Input: part model. Units: mm. Frame: model coordinates. Face numbers are marked on the shaded views. A direction names the side the tool comes from. Coordinates: 2 decimals unless noted, no trailing zeros. Write each loop counter-clockwise with the first axis right and the second up, starting at its lowest first coordinate (ties: lowest second). Pieces come first, ordered by that corner, then holes.
1) Section query D-D (y = -5). Output: boundary loops of the cut face in (x, z).
2) Section query B-B (x = -16.5). Output: boundary loops of the cut face in (y, z) (3 decimals).
3) Section query A-A (z = 0). Output: boundary loops of the cut face in (x, y), then the cut area to 3 significant figures.
4) Line query: L1, parallel to X at y = -50, z = 9.25; L2, parallel to Y at x = -9, z = 0; L3, parallel to X at y = -26, z = 4. Output: solid intervals per line, ascending.
5) Draft query along Z for the marked faces 1, 2 and 3. Return one class per face: pulls with the +Z half, pulls with the -Z half, needs draft (parallel to the pull), parting line crosses it, or undercut.
6) Pin query (flat end, axial travel): pin 1 Ø8 at (y, z) = (10, -2.5) entering from -X; pin 2 Ø12 at (y, z) = (-28.5, 0.5) entering from +X; pin 3 Ø10 at (y, z) = (14.5, 1.5) entering from +X; pin 4 Ø3 at (y, z) = (-20, -3) entering from -X. Return the tip coordinate at first contact, or that it passes through.
7) Set-up query: the marked faces 4, 5 and 6. Return all of +Z, -Z, +X, -X, +Y, -Y with unobstructed straight access to the full face (end or side cutting, diameter ignored); none if empty.
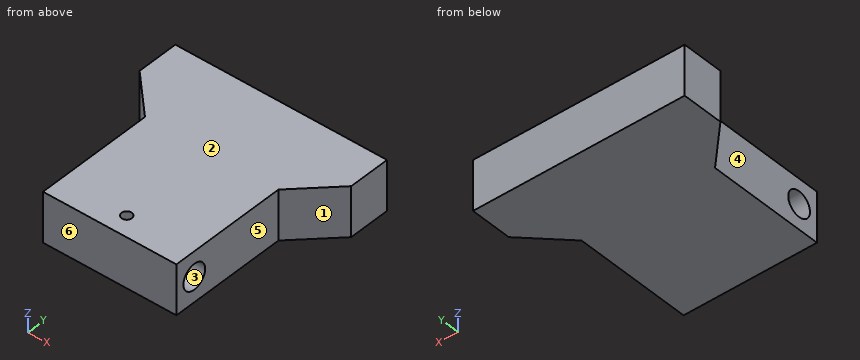
Autodesk Inventor part; units mm, degrees
ref_plane "YZ Plane" through (0, 0, 0) normal (1, 0, 0) x (0, 1, 0)
ref_plane "XZ Plane" through (0, 0, 0) normal (0, 1, 0) x (-1, 0, 0)
ref_plane "XY Plane" through (0, 0, 0) normal (0, 0, 1) x (1, 0, 0)
sketch "Esboço1" plane through (0, 0, 0) normal (0, 0, 1) x (1, 0, 0)
  line L0 (0, 36.3068) -> (0, -8.6932) construction
  circle A0 centre (0, -8.6932) radius 68 construction
  line L1 (0, 36.3068) -> (50.9804, 36.3068)
  line L2 (50.9804, 36.3068) -> (50.9804, 16.3068)
  line L3 (50.9804, 16.3068) -> (32.1355, -2.5381)
  line L4 (32.1355, -2.5381) -> (32.1355, -59.5381)
  line L5 (32.1355, -59.5381) -> (0, -59.5381)
  line L6 (0, -76.6932) -> (0, 59.3068) construction
  line L7 (0, 36.3068) -> (-50.9804, 36.3068)
  line L8 (-50.9804, 36.3068) -> (-50.9804, 16.3068)
  line L9 (-50.9804, 16.3068) -> (-32.1355, -2.5381)
  line L10 (-32.1355, -2.5381) -> (-32.1355, -59.5381)
  line L11 (-32.1355, -59.5381) -> (0, -59.5381)
  point P0 (0, 0)
  dimension "d1" = 45
  dimension "d2" = 136
  dimension "d3" = 20
  dimension "d4" = 135
  dimension "d5" = 57
  dimension "d7" = 50.9804
  dimension "d41" = 32.1355
extrude "Extrusão1" add sketch "Esboço1" along normal mid plane 24
sketch "Esboço2" plane through (-32.1355, -59.5381, 12) normal (-1, 0, 0) x (0, 0, 1)
  line L0 (0, 0) -> (-24, 0) construction
  line L1 (-12, 0) -> (-12, 10) construction
  circle A0 centre (-12, 10) radius 6.075
  point P0 (-12, 59.5381)
  dimension "d10" = 10
  dimension "d11" = 12.15
hole "Furo1" at (-32.1355, -49.5381, 0) direction (1, 0, 0) diameter 12.15 end through all
sketch "Esboço3" plane through (0, 0, 12) normal (0, 0, 1) x (1, 0, 0)
  line L0 (0, 0) -> (0, -50) construction
  dimension "d42" = 50
hole "Furo2" at (0, -50, 12) direction (0, 0, -1) diameter 4.917 depth 10 tip angle 118
properties part number "suporte_guia_central" material "Alumínio 6061"
Answer:
1. outline: (-32.14, -12) - (32.14, -12) - (32.14, 12) - (-32.14, 12) - close
2. outline: (-59.538, -12) - (36.307, -12) - (36.307, 12) - (-59.538, 12) - close; hole circle Ø12.15 at (-49.538, 0)
3. outline: (-50.98, 16.31) - (-32.14, -2.54) - (-32.14, -43.46) - (32.14, -43.46) - (32.14, -2.54) - (50.98, 16.31) - (50.98, 36.31) - (-50.98, 36.31) - close; (-32.14, -59.54) - (32.14, -59.54) - (32.14, -55.61) - (-32.14, -55.61) - close
3. area: 6,490 mm2
4. L1: x = -32.14 to -2.46, 2.46 to 32.14
4. L2: y = -59.54 to -55.61, -43.46 to 36.31
4. L3: x = -32.14 to 32.14
5. face 1: needs draft
5. face 2: pulls with the +Z half
5. face 3: undercut
6. pin 1: stops at x = -48.67
6. pin 2: stops at x = 32.14
6. pin 3: stops at x = 50.98
6. pin 4: stops at x = -32.14
7. face 4: +Z, -Z, -X, -Y
7. face 5: +Z, -Z, +X, -Y
7. face 6: +Z, -Z, +X, -X, -Y
